Verification items for the finished model (mm, model axes). Face numbers are marked on the shaded views. A direction names the side the tool comes from. Give positions to 0.01 mm unless a question says otherwise; leave off trailing zeros. Loops run counter-clockwise (first coordinate to the right, second up) from the corner with the lowest first, then second, coordinate; pieces in that order, holes last. Notation, with made-up numbers: (-13, 61) - (-5, 61) arc R10 cw to (-5, 70) - close; hole circle Ø9 at (7.25, 53). An arc over 180 degrees is marked (long way). Use one line per item in the form item = value.
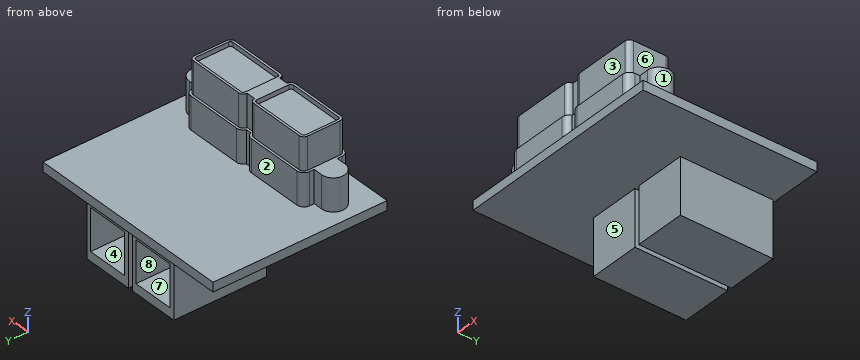
```python
from build123d import *

# Parameters (mm, degrees)
SKETCH1_W           = 45
SKETCH1_H           = 37.5
BOSS_EXTRUDE1_DEPTH = 2
SKETCH2_W           = 40
SKETCH2_H           = 13
BOSS_EXTRUDE2_DEPTH = 7
BOSS_EXTRUDE3_DEPTH = 7
FILLET1_R           = 1
CUT_EXTRUDE1_DEPTH  = 1
SKETCH5_W           = 41
SKETCH5_H           = 14
CUT_EXTRUDE2_DEPTH  = 7
SKETCH6_W           = 11
SKETCH6_H           = 20
BOSS_EXTRUDE5_DEPTH = 12
SKETCH7_W           = 9
SKETCH7_H           = 9
CUT_EXTRUDE3_DEPTH  = 12


with BuildPart() as part:
    # Sketch1 → Boss-Extrude1 (new body)
    with BuildSketch(Plane.XY):
        Rectangle(SKETCH1_W, SKETCH1_H)
    extrude(amount=BOSS_EXTRUDE1_DEPTH)

    # Sketch2 → Boss-Extrude2 (add)
    with BuildSketch(Plane.XY.offset(2)):
        with Locations((0, -11.25)):
            Rectangle(SKETCH2_W, SKETCH2_H)
    extrude(amount=BOSS_EXTRUDE2_DEPTH)

    # Sketch3 → Boss-Extrude3 (add)
    with BuildSketch(Plane.XY.offset(9)):
        Polygon((-1, -7.75), (-1, -6.75), (-15, -6.75), (-15, -15.75), (-1, -15.75), (-1, -14.75), (1, -14.75), (1, -15.75), (15, -15.75), (15, -6.75), (1, -6.75), (1, -7.75), align=None)
    extrude(amount=BOSS_EXTRUDE3_DEPTH)

    # Fillet1
    fillet1_edges = [part.edges().sort_by_distance(p)[0] for p in [
        (-15, -15.75, 12.5),
        (-1, -15.75, 12.5),
        (1, -15.75, 12.5),
        (-15, -6.75, 12.5),
        (15, -15.75, 12.5),
        (15, -6.75, 12.5),
        (1, -6.75, 12.5),
        (-1, -6.75, 12.5),
    ]]
    fillet(fillet1_edges, radius=FILLET1_R - 0.0001)  # a hair under: the kernel refuses the full size

    # Sketch4 → Cut-Extrude1 (cut)
    with BuildSketch(Plane.XY.offset(16)):
        with BuildLine():
            Line((-1.5, -14.75), (-1.5, -7.75))
            ThreePointArc((-1.5, -7.75), (-1.646446609, -7.396446609), (-2, -7.25))
            Line((-2, -7.25), (-14, -7.25))
            ThreePointArc((-14, -7.25), (-14.353553391, -7.396446609), (-14.5, -7.75))
            Line((-14.5, -7.75), (-14.5, -14.75))
            ThreePointArc((-14.5, -14.75), (-14.353553391, -15.103553391), (-14, -15.25))
            Line((-14, -15.25), (-2, -15.25))
            ThreePointArc((-2, -15.25), (-1.646446609, -15.103553391), (-1.5, -14.75))
        make_face()
        with BuildLine():
            Line((1.5, -7.75), (1.5, -14.75))
            ThreePointArc((1.5, -14.75), (1.646446609, -15.103553391), (2, -15.25))
            Line((2, -15.25), (14, -15.25))
            ThreePointArc((14, -15.25), (14.353553391, -15.103553391), (14.5, -14.75))
            Line((14.5, -14.75), (14.5, -7.75))
            ThreePointArc((14.5, -7.75), (14.353553391, -7.396446609), (14, -7.25))
            Line((14, -7.25), (2, -7.25))
            ThreePointArc((2, -7.25), (1.646446609, -7.396446609), (1.5, -7.75))
        make_face()
    extrude(amount=-CUT_EXTRUDE1_DEPTH, mode=Mode.SUBTRACT)

    # Sketch5 → Cut-Extrude2 (cut)
    with BuildSketch(Plane.XY.offset(9)):
        with Locations((0, -11.25)):
            Rectangle(SKETCH5_W, SKETCH5_H)
        with BuildLine():
            Line((-17.5, -8.75), (-15.5, -8.75))
            Line((-15.5, -8.75), (-15.5, -7.75))
            ThreePointArc((-15.5, -7.75), (-15.060660172, -6.689339828), (-14, -6.25))
            Line((-14, -6.25), (-2, -6.25))
            ThreePointArc((-2, -6.25), (-1.133974596, -6.525255129), (-0.585786438, -7.25))
            Line((-0.585786438, -7.25), (0.585786438, -7.25))
            ThreePointArc((0.585786438, -7.25), (1.133974596, -6.525255129), (2, -6.25))
            Line((2, -6.25), (14, -6.25))
            ThreePointArc((14, -6.25), (15.060660172, -6.689339828), (15.5, -7.75))
            Line((15.5, -7.75), (15.5, -8.75))
            Line((15.5, -8.75), (17.5, -8.75))
            ThreePointArc((17.5, -8.75), (20, -11.25), (17.5, -13.75))
            Line((17.5, -13.75), (15.5, -13.75))
            Line((15.5, -13.75), (15.5, -14.75))
            ThreePointArc((15.5, -14.75), (15.060660172, -15.810660172), (14, -16.25))
            Line((14, -16.25), (2, -16.25))
            ThreePointArc((2, -16.25), (1.133974596, -15.974744871), (0.585786438, -15.25))
            Line((0.585786438, -15.25), (-0.585786438, -15.25))
            ThreePointArc((-0.585786438, -15.25), (-1.133974596, -15.974744871), (-2, -16.25))
            Line((-2, -16.25), (-14, -16.25))
            ThreePointArc((-14, -16.25), (-15.060660172, -15.810660172), (-15.5, -14.75))
            Line((-15.5, -14.75), (-15.5, -13.75))
            Line((-15.5, -13.75), (-17.5, -13.75))
            ThreePointArc((-17.5, -13.75), (-20, -11.25), (-17.5, -8.75))
        make_face(mode=Mode.SUBTRACT)
    extrude(amount=-CUT_EXTRUDE2_DEPTH, mode=Mode.SUBTRACT)

    # Sketch6 → Boss-Extrude5 (add)
    with BuildSketch(Plane(origin=(0, 0, 0), x_dir=(-1, 0, 0), z_dir=(0, 0, -1))):
        with Locations((-6, 8.25)):
            Rectangle(SKETCH6_W, SKETCH6_H)
        with Locations((6, 8.25)):
            Rectangle(SKETCH6_W, SKETCH6_H)
    extrude(amount=BOSS_EXTRUDE5_DEPTH)

    # Sketch7 → Cut-Extrude3 (cut)
    with BuildSketch(Plane(origin=(0, 18.25, 0), x_dir=(1, 0, 0), z_dir=(0, 1, 0))):
        with Locations((-6, 5.5)):
            Rectangle(SKETCH7_W, SKETCH7_H)
        with Locations((6, 5.5)):
            Rectangle(SKETCH7_W, SKETCH7_H)
    extrude(amount=-CUT_EXTRUDE3_DEPTH, mode=Mode.SUBTRACT)


solid = part.part
```
1. Scan lines: probe 1 along X at (y, z) = (16.5, -7); probe 2 along X at (y, z) = (3, -6.5); probe 3 along Z at (x, y) = (8, -12). Record each from-to range of solid material in increasing order.
Result set:
probe_1 = -11.5 to -10.5, -1.5 to -0.5, 0.5 to 1.5, 10.5 to 11.5
probe_2 = -11.5 to -0.5, 0.5 to 11.5
probe_3 = 0 to 15
2. Section check D-D, the plane y = -11.25. Record the cut outline in (x, z).
Result set:
outline = (-22.5, 0) - (22.5, 0) - (22.5, 2) - (20, 2) - (20, 9) - (15, 9) - (15, 16) - (14.5, 16) - (14.5, 15) - (1.5, 15) - (1.5, 16) - (-1.5, 16) - (-1.5, 15) - (-14.5, 15) - (-14.5, 16) - (-15, 16) - (-15, 9) - (-20, 9) - (-20, 2) - (-22.5, 2) - close
3. Tool access check on the marked faces 1, 2, 3 and 4. Record the directions out of +Z, -Z, +X, -X, +Y, -Y that give a thin tool (end or side, any length) a straight path to the whole face; none if there is none.
Result set:
face_1 = +Z, +X
face_2 = +Z, +X, -X, +Y
face_3 = +Z, +X, -X, -Y
face_4 = +Y
4. Section check C-C, the plane x = -5. Record the cut outline in (y, z).
Result set:
outline = (-18.75, 0) - (-1.75, 0) - (-1.75, -12) - (18.25, -12) - (18.25, -10) - (6.25, -10) - (6.25, -1) - (18.25, -1) - (18.25, 0) - (18.75, 0) - (18.75, 2) - (-6.25, 2) - (-6.25, 9) - (-6.75, 9) - (-6.75, 16) - (-7.25, 16) - (-7.25, 15) - (-15.25, 15) - (-15.25, 16) - (-15.75, 16) - (-15.75, 9) - (-16.25, 9) - (-16.25, 2) - (-18.75, 2) - close
5. Section check A-A, the plane y = 7. Record the cut outline in (x, z), then the cut area to 3 significant figures.
Result set:
outline = (-22.5, 0) - (-11.5, 0) - (-11.5, -12) - (-0.5, -12) - (-0.5, 0) - (0.5, 0) - (0.5, -12) - (11.5, -12) - (11.5, 0) - (22.5, 0) - (22.5, 2) - (-22.5, 2) - close; hole (-10.5, -10) - (-1.5, -10) - (-1.5, -1) - (-10.5, -1) - close; hole (1.5, -10) - (10.5, -10) - (10.5, -1) - (1.5, -1) - close
area = 192 mm²
6. Draft check along X on the marked faces 5, 6, 7 and 8. Enter one of: released by +X, released by -X, zero draft, split by the parting line, or undercut.
Result set:
face_5 = zero draft
face_6 = released by +X
face_7 = undercut
face_8 = undercut
7. Section check B-B, the plane z = -1.75. Record the cut outline in (x, y), then the cut area to 3 significant figures.
Result set:
outline = (-11.5, -1.75) - (-0.5, -1.75) - (-0.5, 18.25) - (-1.5, 18.25) - (-1.5, 6.25) - (-10.5, 6.25) - (-10.5, 18.25) - (-11.5, 18.25) - close; (0.5, -1.75) - (11.5, -1.75) - (11.5, 18.25) - (10.5, 18.25) - (10.5, 6.25) - (1.5, 6.25) - (1.5, 18.25) - (0.5, 18.25) - close
area = 224 mm²
8. Depth check by flat-ended pin: pin 1 Ø1.1 at (x, z) = (8.5, 15.5) entering from -Y; pin 2 Ø5.5 at (x, z) = (-3.5, -5.5) entering from -Y; pin 3 Ø7.5 at (x, z) = (10, 14) entering from +Y. Enter the tip coordinate at first touch or a pass-through.
Result set:
pin_1 = -15.75
pin_2 = -1.75
pin_3 = -6.75
